from build123d import *

# Parameters (mm, degrees)
CROQUIS1_W              = 60
CROQUIS1_H              = 60
CROQUIS1_R              = 10
SALIENTE_EXTRUIR1_DEPTH = 80
CROQUIS2_R              = 4
CORTAR_EXTRUIR1_DEPTH   = 20


with BuildPart() as part:
    # Croquis1 → Saliente-Extruir1 (new body)
    with BuildSketch(Plane(origin=(0, 0, 0), x_dir=(1, 0, 0), z_dir=(0, 1, 0))):
        Rectangle(CROQUIS1_W, CROQUIS1_H)
        with Locations(Location((0, 0, 0), (0, 0, 270))):
            Circle(CROQUIS1_R, mode=Mode.SUBTRACT)
    extrude(amount=SALIENTE_EXTRUIR1_DEPTH)

    # Croquis2 → Cortar-Extruir1 (cut)
    with BuildSketch(Plane.XY.offset(30)):
        with Locations((-15, 60)):
            Circle(CROQUIS2_R)
        with Locations((15, 60)):
            Circle(CROQUIS2_R)
        with Locations((-15, 20)):
            Circle(CROQUIS2_R)
        with Locations((15, 20)):
            Circle(CROQUIS2_R)
    extrude(amount=-CORTAR_EXTRUIR1_DEPTH, mode=Mode.SUBTRACT)


solid = part.part
The model under review builds one solid part; all positions refer to its coordinate system, in mm. A direction names the side the tool comes from. Round coordinates to 2 decimals unless told otherwise and drop trailing zeros. Loops run counter-clockwise (first coordinate to the right, second up) from the corner with the lowest first, then second, coordinate; pieces in that order, holes last. Notation, with made-up numbers: (12.5, 82.5) -> (38.5, 82.5) arc R21 cw to (38.5, 88.5) -> close; hole circle Ø8 at (82.5, 77.25). An arc over 180 degrees is marked (long way). One line per question, with ' | ' between items. Start each with the question number.
Item 1: Wall thickness on line 1 along Y through (x, z) = (15, 14); line 2 along X through (y, z) = (51, 0); line 3 along Y through (x, z) = (11.5, 25): over which ranges is each line inside the solid? List them lowest first. Write a range as [from, to].
Item 2: Add section B-B, the plane z = 0. Write out the cut boundary in (x, y).
Item 3: For pin 1 (5 mm diameter, centred on x = 15, y = 20, fed in from +Z); pin 2 (12 mm diameter, centred on x = -14.5, z = 17.5, fed in from -Y); pin 3 (16 mm diameter, centred on x = 0, z = 0, fed in from +Y), all flat-tipped, find the tip position at first contact; note any pin that passes through.
Item 4: Machinability: for faces 1 (the face through (0, 39, -30)), 2 (the face through (-15.867, 56.095, 20.14)), which of the approach directions +Z, -Z, +X, -X, +Y, -Y give a long, thin tool a straight path to every point of the face, cutting with its end or side? Answer none if there is none.
Item 5: Draft analysis for pull direction X (two halves, no side actions). For faces 3 (the face through (12.05, 22.7, 20.14)), 4 (the face through (-14, 80, 0)), 5 (the face through (-30, 39, 0)), state which applies: +X half, -X half, draft (parallel to the pull), parting line (faces both ways), or undercut.
Item 6: Add section D-D, the plane x = 15. Write out the cut boundary in (y, z), then the cut area to 3 significant figures.
Item 7: Add section A-A, the plane x = -6. Write out the cut boundary in (y, z).
Item 8: Add section C-C, the plane y = 44. Write out the cut boundary in (x, z), then the cut area to 3 significant figures.
Return value:
1) line 1: y = [0, 16], [24, 56], [64, 80] | line 2: x = [-30, -10], [10, 30] | line 3: y = [0, 18.06], [21.94, 58.06], [61.94, 80]
2) outline: (-30, 0) -> (-10, 0) -> (-10, 80) -> (-30, 80) -> close; (10, 0) -> (30, 0) -> (30, 80) -> (10, 80) -> close
3) pin 1: stops at z = 10 | pin 2: stops at y = 0 | pin 3: passes through
4) face 1: -Z, +X, -X, +Y, -Y | face 2: +Z
5) face 3: undercut | face 4: draft | face 5: -X half
6) outline: (0, -30) -> (80, -30) -> (80, 30) -> (64, 30) -> (64, 10) -> (56, 10) -> (56, 30) -> (24, 30) -> (24, 10) -> (16, 10) -> (16, 30) -> (0, 30) -> close | area: 4,480 mm2
7) outline: (0, -30) -> (80, -30) -> (80, -8) -> (0, -8) -> close; (0, 8) -> (80, 8) -> (80, 30) -> (0, 30) -> close
8) outline: (-30, -30) -> (30, -30) -> (30, 30) -> (-30, 30) -> close; hole circle Ø20 at (0, 0) | area: 3,290 mm2
